Print and shaded views of the part. All mm, measured from the part's lowest x, y and z. A direction names the side the tool comes from. Coordinates: 2 decimals unless noted, no trailing zeros. Order: outer loops, then holes, each group sorted by start corner. A loop starts at its lowest first (then second) coordinate and runs counter-clockwise, first axis right, second up. Notation, with made-up numbers: M 63,-35.5 L 79,-35.5 A34 ccw 79,-0.5 Z; hole C 57.25,56 d11. An arc over 180 degrees is marked long. One line per item, written item: value.
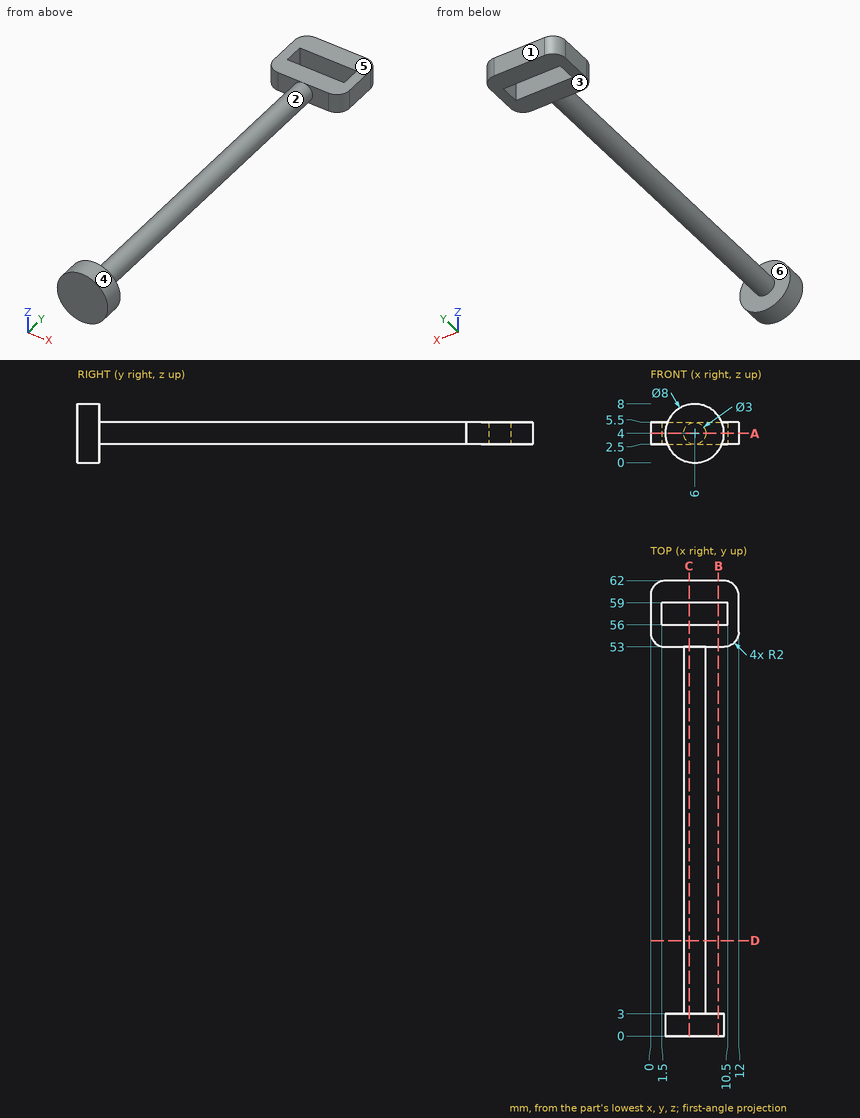
Q1. Slice it at C-C (x = 5.25). List the corners of the cut face in (y, z), plus the area to 3 significant figures.
Recorded:
outline: M 0,0.07 L 3,0.07 L 3,2.7 L 53,2.7 L 53,2.5 L 56,2.5 L 56,5.5 L 53,5.5 L 53,5.3 L 3,5.3 L 3,7.93 L 0,7.93 Z; M 59,2.5 L 62,2.5 L 62,5.5 L 59,5.5 Z
area: 171 mm^2
Q2. Mould opens along Y. For the marked faces 1, 2 and 3 say: released by +Y, released by -Y, zero draft, split by the parting line, or undercut.
Recorded:
face 1: released by +Y
face 2: undercut
face 3: zero draft
Q3. Drill centre lines: line 1 along Y through (x, z) = (9.25, 2.75); line 2 along Y through (x, z) = (6, 1); line 3 along Y through (x, z) = (10.25, 5). Where is each one in solid material? Low to high.
Recorded:
line 1: y = 0 to 3, 53 to 56, 59 to 62
line 2: y = 0 to 3
line 3: y = 53.02 to 56, 59 to 61.98
Q4. Which spindle directions (+Z, -Z, +X, -X, +Y, -Y) get a long thin tool onto all of the face, cutting with end or side? Do the marked faces 4, 5 and 6. Say none if no direction does.
Recorded:
face 4: -Y
face 5: +Z, +X, -X, +Y
face 6: none
Q5. Slice it at B-B (x = 9.25). List the corners of the cut face in (y, z).
Recorded:
outline: M 0,1.67 L 3,1.67 L 3,6.33 L 0,6.33 Z; M 53,2.5 L 56,2.5 L 56,5.5 L 53,5.5 Z; M 59,2.5 L 62,2.5 L 62,5.5 L 59,5.5 Z
Q6. Pin check, flat tips, straight feed: pin 1 Ø1 at (x, y) = (7.5, 10.5) entering from -Z; pin 2 Ø5 at (x, y) = (6.5, 17.5) entering from -Z. Stop position of each tip, or through.
Recorded:
pin 1: stops at z = 2.88
pin 2: stops at z = 2.5
Q7. Slice it at D-D (y = 13). List the corners of the cut face in (x, z), plus the area to 3 significant figures.
Recorded:
outline: C 6,4 d3
area: 7.07 mm^2
Q8. Slice it at A-A (z = 4). List the corners of the cut face in (x, y).
Recorded:
outline: M 0,55 A2 ccw 2,53 L 4.5,53 L 4.5,3 L 2,3 L 2,0 L 10,0 L 10,3 L 7.5,3 L 7.5,53 L 10,53 A2 ccw 12,55 L 12,60 A2 ccw 10,62 L 2,62 A2 ccw 0,60 Z; hole M 1.5,56 L 10.5,56 L 10.5,59 L 1.5,59 Z
